Verification items for the finished model (mm, model axes). Face numbers are marked on the shaded views. A direction names the side the tool comes from. Give positions to 0.01 mm unless a question says otherwise; leave off trailing zeros. Loops run counter-clockwise (first coordinate to the right, second up) from the corner with the lowest first, then second, coordinate; pieces in that order, holes last. Notation, with made-up numbers: M 5,70 L 14,70 A15 ccw 14,78 Z; hole C -31,7 d2. An arc over 180 degrees is marked long. Answer in a Markdown table with one row per item.
```python
from build123d import *

# Parameters (mm, degrees)
F0_W     = 76.2
F0_H     = 76.2
F1_DEPTH = 3
F2_W     = 76.2
F2_H     = 76.2
F2_W_2   = 70.2
F2_H_2   = 70.2
F3_DEPTH = 38.1
F4_R     = 12.7
F5_DEPTH = 12.7
F6_R     = 3.175
F7_DEPTH = 25.4


with BuildPart() as f1:
    # F0 (on Top) → F1 (new body)
    with BuildSketch(Plane.XY):
        with Locations((-38.1, 38.1)):
            Rectangle(F0_W, F0_H)
    extrude(amount=F1_DEPTH)

    # F2 (on face) → F3 (join)
    with BuildSketch(Plane.XY.offset(3)):
        with Locations((-38.1, 38.1)):
            Rectangle(F2_W, F2_H)
        with Locations((-38.1, 38.1)):
            Rectangle(F2_W_2, F2_H_2, mode=Mode.SUBTRACT)
    extrude(amount=F3_DEPTH)

    # F4 (on face) → F5 (join)
    with BuildSketch(Plane.XY.offset(3)):
        with Locations((-38.1, 38.1)):
            Circle(F4_R)
    extrude(amount=F5_DEPTH)

    # F6 (on face) → F7 (join)
    with BuildSketch(Plane.XY.offset(15.7)):
        with Locations((-38.1, 38.1)):
            Circle(F6_R)
    extrude(amount=F7_DEPTH)


solid = f1.part
```
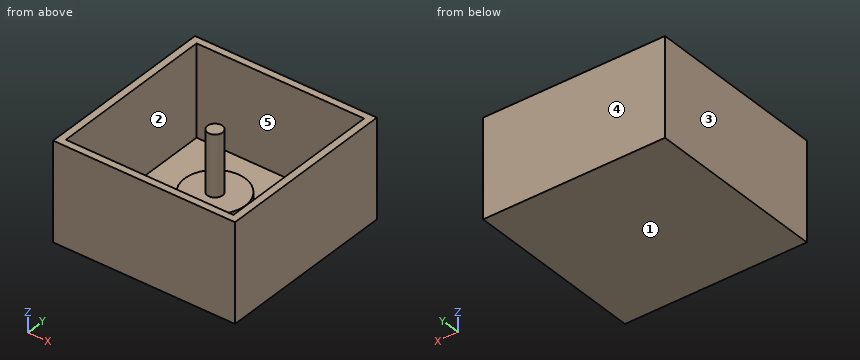
Item 1: Sectioned sample at B-B (y = 38.1). Record the cut outline in (x, z) (3 decimals).
Reported:
| item | result |
|---|---|
| outline | M -76.2,0 L 0,0 L 0,41.1 L -3,41.1 L -3,3 L -25.4,3 L -25.4,15.7 L -34.925,15.7 L -34.925,41.1 L -41.275,41.1 L -41.275,15.7 L -50.8,15.7 L -50.8,3 L -73.2,3 L -73.2,41.1 L -76.2,41.1 Z |
Item 2: Sectioned sample at C-C (z = 18). Record the cut outline in (x, y) (3 decimals), and give its area (3 significant figures).
Reported:
| item | result |
|---|---|
| outline | M -76.2,0 L 0,0 L 0,76.2 L -76.2,76.2 Z; C -38.1,38.1 d6.35; hole M -73.2,3 L -3,3 L -3,73.2 L -73.2,73.2 Z |
| area | 910 mm^2 |
Item 3: Sectioned sample at A-A (z = 5.5). Record the cut outline in (x, y).
Reported:
| item | result |
|---|---|
| outline | M -76.2,0 L 0,0 L 0,76.2 L -76.2,76.2 Z; C -38.1,38.1 d25.4; hole M -73.2,3 L -3,3 L -3,73.2 L -73.2,73.2 Z |
Item 4: Release check for a two-part mould opening along X. For the marked faces 1, 2 and 3 record: released by +X, released by -X, zero draft, split by the parting line, or undercut.
Reported:
| item | result |
|---|---|
| face 1 | zero draft |
| face 2 | undercut |
| face 3 | released by -X |
Item 5: Go/stop test with a flat-tipped pin: pin 1 (2 mm diameter, centred on x = -67.5, y = 25, fed in from +Z). Record where the tip stops, or that it passes through.
Reported:
| item | result |
|---|---|
| pin 1 | stops at z = 3 |
Item 6: Sectioned sample at D-D (x = -64). Record the cut outline in (y, z), and give its area (3 significant figures).
Reported:
| item | result |
|---|---|
| outline | M 0,0 L 76.2,0 L 76.2,41.1 L 73.2,41.1 L 73.2,3 L 3,3 L 3,41.1 L 0,41.1 Z |
| area | 457 mm^2 |
Item 7: Scan lines: L1, parallel to Y at x = -5.5, z = 37; L2, parallel to X at y = 17, z = 27.5; L3, parallel to X at y = 36.5, z = 17.5. Record each from-to range of solid material in increasing order. Write a range as [from, to].
Reported:
| item | result |
|---|---|
| L1 | y = [0, 3], [73.2, 76.2] |
| L2 | x = [-76.2, -73.2], [-3, 0] |
| L3 | x = [-76.2, -73.2], [-40.84, -35.36], [-3, 0] |
Item 8: Tool access check on the marked faces 4 and 5. Record the directions out of +Z, -Z, +X, -X, +Y, -Y that give a thin tool (end or side, any length) a straight path to the whole face; none if there is none.
Reported:
| item | result |
|---|---|
| face 4 | +Z, -Z, +X, -X, +Y |
| face 5 | +Z |
